Check sheet for the drawn part. Datum: minimum x, y, z corner. Units: mm. A direction names the side the tool comes from. Give positions to 0.01 mm unless a question says otherwise; leave off trailing zeros. Write each loop counter-clockwise with the first axis right and the second up, starting at its lowest first coordinate (ties: lowest second). Pieces come first, ordered by that corner, then holes. Notation, with made-up numbers: (86.5, 15.5) - (122.5, 15.5) arc R14 ccw to (122.5, 22.5) - close; hole circle Ø1 at (-12.5, 4). An arc over 180 degrees is marked (long way). Return JSON: item names as keys, results as strings. Group by question number.
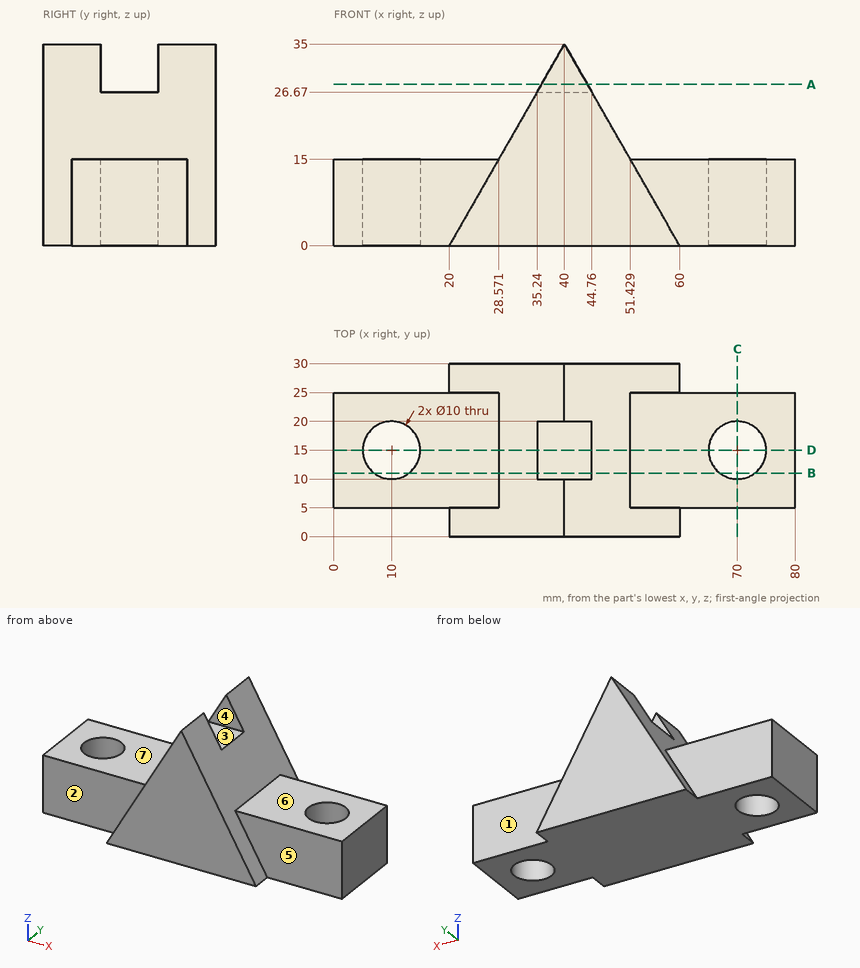
Item 1: Mould release check, pull along Y, two halves, no side actions. Record for the marked faces 1, 2, 3 and 4: +Y half, -Y half, draft (parallel to the pull), parting line (faces both ways), or undercut.
Item 2: Section check A-A on z = 28. Record the cut outline in (x, y).
Item 3: Material ranges on line 1 along Y through (x, z) = (70, 7); line 2 along Z through (x, y) = (14, 8.75); line 3 along Y through (x, z) = (36.5, 27), recorded low to high. Write a range as from..to.
Item 4: Section check D-D on y = 15. Record the cut outline in (x, z).
Item 5: Section check B-B on y = 11. Record the cut outline in (x, z), plus the area to 3 significant figures.
Item 6: Section check C-C on x = 70. Record the cut outline in (y, z), plus the area to 3 significant figures.
Item 7: Depth check by flat-ended pin: pin 1 (12 mm diameter, centred on x = 71, z = 6, fed in from -Y); pin 2 (6 mm diameter, centred on x = 18.5, y = 13.5, fed in from +Z); pin 3 (2 mm diameter, centred on y = 18, z = 17.5, fed in from +X); pin 4 (8 mm diameter, centred on x = 10, y = 15, fed in from +Z). Enter the tip coordinate at first touch or a pass-through.
Item 8: Access from +Z, -Z, +X, -X, +Y, -Y to the whole of each face (thin tool, end or side, straight path). Record for the marked faces 5, 6 and 7.
Reply:
{
 "1": {"face 1": "+Y half", "face 2": "-Y half", "face 3": "undercut", "face 4": "undercut"},
 "2": {"outline": "(36, 0) - (44, 0) - (44, 10) - (36, 10) - close; (36, 20) - (44, 20) - (44, 30) - (36, 30) - close"},
 "3": {"line 1": "5..10, 20..25", "line 2": "0..15", "line 3": "0..10, 20..30"},
 "4": {"outline": "(0, 0) - (5, 0) - (5, 15) - (0, 15) - close; (15, 0) - (65, 0) - (65, 15) - (51.43, 15) - (44.76, 26.67) - (35.24, 26.67) - (28.57, 15) - (15, 15) - close; (75, 0) - (80, 0) - (80, 15) - (75, 15) - close"},
 "5": {"outline": "(0, 0) - (7, 0) - (7, 15) - (0, 15) - close; (13, 0) - (67, 0) - (67, 15) - (51.43, 15) - (44.76, 26.67) - (35.24, 26.67) - (28.57, 15) - (13, 15) - close; (73, 0) - (80, 0) - (80, 15) - (73, 15) - close", "area": "1,210 mm²"},
 "6": {"outline": "(5, 0) - (10, 0) - (10, 15) - (5, 15) - close; (20, 0) - (25, 0) - (25, 15) - (20, 15) - close", "area": "150 mm²"},
 "7": {"pin 1": "y = 5", "pin 2": "z = 15", "pin 3": "x = 50.57", "pin 4": "through"},
 "8": {"face 5": "+Z, +X, -Y", "face 6": "+Z, +X, +Y, -Y", "face 7": "+Z, -X, +Y, -Y"}
}
